Input: dimensioned drawing with shaded views. Units: mm. Origin: part minimum x, y, z. Round coordinates to 2 decimals unless told otherwise and drop trailing zeros. Loops run counter-clockwise (first coordinate to the right, second up) from the corner with the lowest first, then second, coordinate; pieces in that order, holes last. Notation, with made-up numbers: M 27,-32 L 60,-32 A21 cw 60,-5 Z; hole C -27.75,57.5 d9. An arc over 180 degrees is marked long. Use one line per item in the form item = value. Start each with the question number.
Q1. Section query A-A, the plane z = 1.7. Output: boundary loops of the cut face in (x, y) (1 decimal).
Q2. First-contact query: P1, Ø6, axis at x = 20, y = 20, coming from the -Z side; P2, Ø1.5, axis at y = 70.5, z = 2, coming from the +X side; P3, Ø1.5, axis at x = 53.5, z = 2, coming from the +Y side; P4, Ø0.9, axis at x = 54, z = 1, coming from the -Y side. Flat tips, straight axial feed; report the tip coordinate or a pass-through.
Q3. Section query D-D, the plane x = 41. Output: boundary loops of the cut face in (y, z) (1 decimal), and give its area (3 significant figures).
Q4. Ray query, line 1 along X through (y, z) = (20, 1.35); line 2 along Y through (x, z) = (20, 1.65) (1 decimal); line 3 along Y through (x, z) = (21, 1.55) (1 decimal). Return the intervals inside material, ascending.
Q5. Section query B-B, the plane y = 20. Output: boundary loops of the cut face in (x, z), and give its area (3 significant figures).
Q6. Section query C-C, the plane x = 20. Output: boundary loops of the cut face in (y, z).
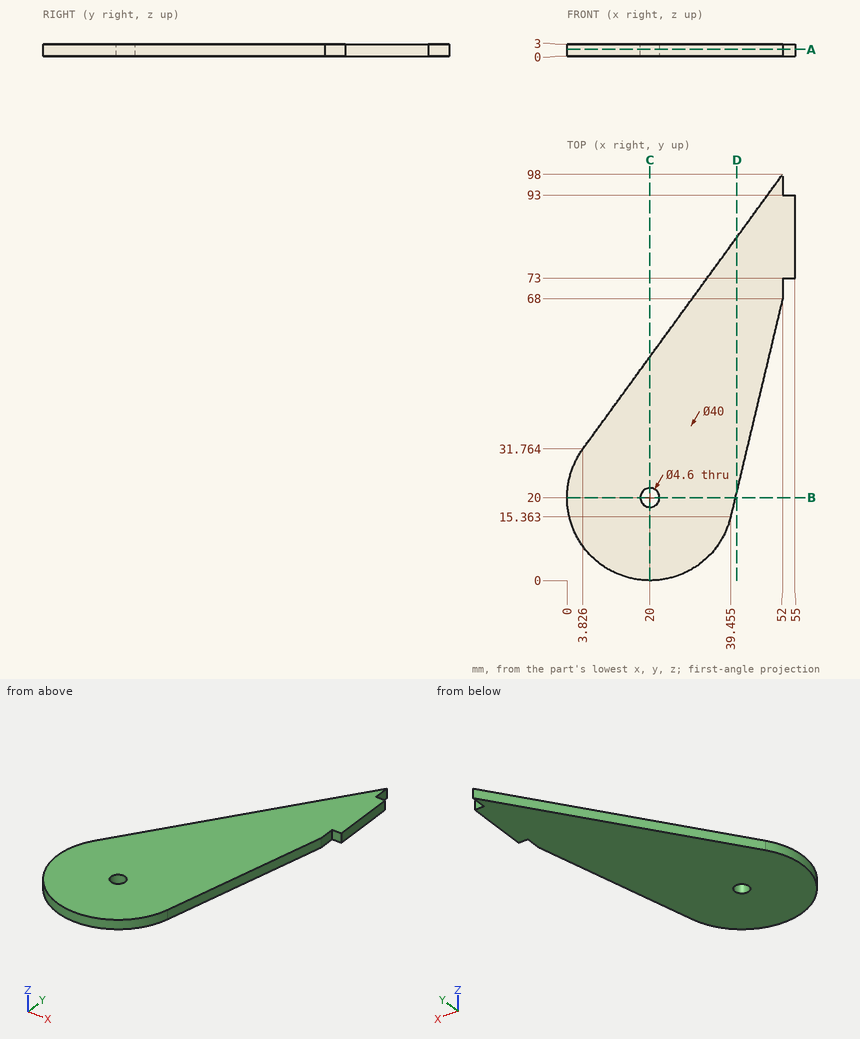
Results found:
q1.outline = M 3.8,31.8 A20 ccw long 39.5,15.4 L 52,68 L 52,73 L 55,73 L 55,93 L 52,93 L 52,98 Z; hole C 20,20 d4.6
q2.P1 = 0
q2.P2 = 52
q2.P3 = 93
q2.P4 = 73
q3.outline = M 21.8,0 L 82.9,0 L 82.9,3 L 21.8,3 Z
q3.area = 183 mm²
q4.line_1 = 0 to 17.7, 22.3 to 40.56
q4.line_2 = 0 to 17.7, 22.3 to 54
q4.line_3 = 0 to 17.9, 22.1 to 55.4
q5.outline = M 0,0 L 17.7,0 L 17.7,3 L 0,3 Z; M 22.3,0 L 40.56,0 L 40.56,3 L 22.3,3 Z
q5.area = 108 mm²
q6.outline = M 0,0 L 17.7,0 L 17.7,3 L 0,3 Z; M 22.3,0 L 54,0 L 54,3 L 22.3,3 Z
